For this review, use the dimensioned drawing (mm, ordinates from the lowest corner) and the shaded views. Round coordinates to 2 decimals unless told otherwise and drop trailing zeros. Write each loop counter-clockwise with the first axis right and the second up, starting at its lowest first coordinate (ties: lowest second). Pieces come first, ordered by that corner, then holes. Notation, with made-up numbers: M 25.25,73.25 L 50.25,73.25 A28 cw 50.25,101.25 Z; hole C -30.75,3 d9. An arc over 180 degrees is marked long. Answer in a Markdown table with one row per item.
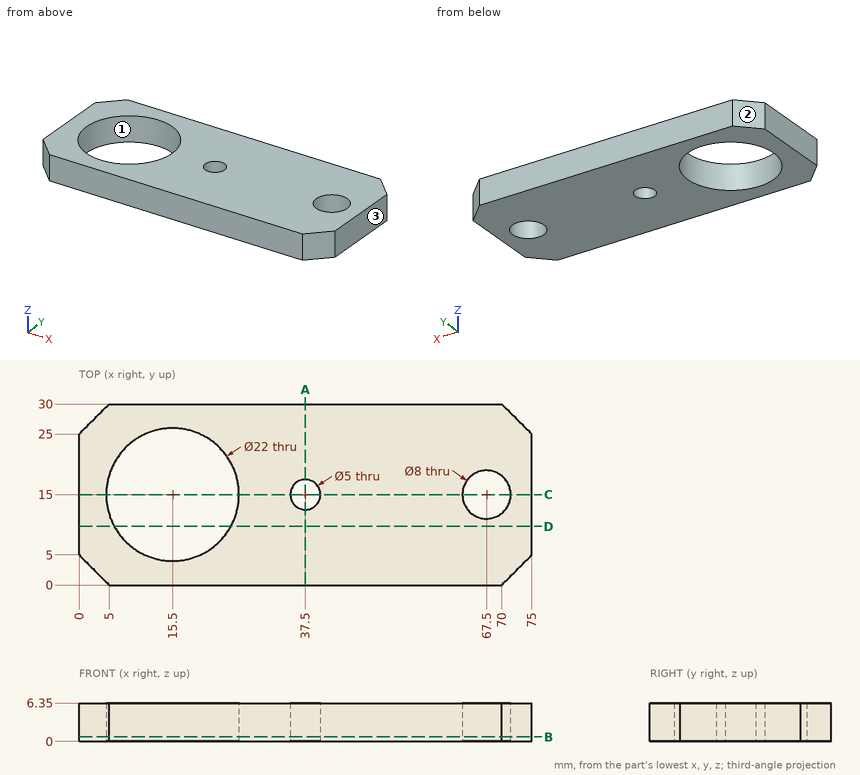
Q1. Take a section at A-A (x = 37.5). State the section outline as (y, z) points, then the cut area to 3 significant figures.
Found:
| item | result |
|---|---|
| outline | M 0,0 L 12.5,0 L 12.5,6.35 L 0,6.35 Z; M 17.5,0 L 30,0 L 30,6.35 L 17.5,6.35 Z |
| area | 159 mm² |
Q2. Take a section at B-B (z = 0.75). State the section outline as (x, y) points, then the cut area to 3 significant figures.
Found:
| item | result |
|---|---|
| outline | M 0,5 L 5,0 L 70,0 L 75,5 L 75,25 L 70,30 L 5,30 L 0,25 Z; hole C 15.5,15 d22; hole C 37.5,15 d5; hole C 67.5,15 d8 |
| area | 1,750 mm² |
Q3. Mouldability with a two-part tool opening along Y and no side actions: class the marked faces 1, 2 and 3 as +Y half, -Y half, draft (parallel to the pull), parting line (faces both ways), or undercut.
Found:
| item | result |
|---|---|
| face 1 | undercut |
| face 2 | +Y half |
| face 3 | draft |
Q4. For probe 1 along Y at (x, z) = (37.5, 4); probe 2 along X at (y, z) = (13.75, 3.5); probe 3 along Y at (x, z) = (15, 1.25), list the stretches that pass through material, from the lowest coordinate up.
Found:
| item | result |
|---|---|
| probe 1 | 0 to 12.5, 17.5 to 30 |
| probe 2 | 0 to 4.57, 26.43 to 35.33, 39.67 to 63.7, 71.3 to 75 |
| probe 3 | 0 to 4.01, 25.99 to 30 |
Q5. Take a section at D-D (y = 9.75). State the section outline as (x, z) points.
Found:
| item | result |
|---|---|
| outline | M 0,0 L 5.83,0 L 5.83,6.35 L 0,6.35 Z; M 25.17,0 L 75,0 L 75,6.35 L 25.17,6.35 Z |
Q6. Take a section at C-C (y = 15). State the section outline as (x, z) points, then the cut area to 3 significant figures.
Found:
| item | result |
|---|---|
| outline | M 0,0 L 4.5,0 L 4.5,6.35 L 0,6.35 Z; M 26.5,0 L 35,0 L 35,6.35 L 26.5,6.35 Z; M 40,0 L 63.5,0 L 63.5,6.35 L 40,6.35 Z; M 71.5,0 L 75,0 L 75,6.35 L 71.5,6.35 Z |
| area | 254 mm² |
